Model file for the job. Use its own axes, mm. A direction names the side the tool comes from. Coordinates: 2 decimals unless noted, no trailing zeros. Order: outer loops, then holes, each group sorted by start corner. A loop starts at its lowest first (then second) coordinate and runs counter-clockwise, first axis right, second up. Notation, with made-up numbers: (64.5, 5.25) -> (73.5, 5.25) arc R12 ccw to (73.5, 10.25) -> close; hole circle Ø10 at (-18.5, 11.5). An arc over 180 degrees is marked (long way). Use CSV: the item, a comma, the result in double quotes. Start each with the question number.
(1) Cut at C-C on x = 21. Write the cut outline in (y, z), plus the area to 3 significant figures.
(2) Pin check, flat tips, straight feed: pin 1 Ø1 at (x, z) = (13.5, 0) entering from -Y; pin 2 Ø0.5 at (x, y) = (0.5, 0.5) entering from +Z; pin 3 Ø3 at (x, y) = (21, -1) entering from +Z; pin 4 Ø1 at (y, z) = (-2, 0.5) entering from +X. Stop position of each tip, or through.
(3) Cut at D-D on x = 33.5. Write the cut outline in (y, z) (3 decimals).
(4) Probe L1, parallel to X at y = -1.5, z = 0.15; L2, parallel to X at y = 1.7, z = 0.35; L3, parallel to Y at x = 20, z = 0.15 (3 decimals). List the from-to ranges inside material, lowest first.
(5) Cut at B-B on z = 0. Write the cut outline in (x, y) (3 decimals).
(6) Pull direction Z, two halves, no side cores. Call faces 1 (the flat face through (32, 2, 0)), 2 (the cylindrical face through (0.99, -0.65, 2.93)), 3 (the flat face through (0.5, 0, 1)): pulls with the +Z half, pulls with the -Z half, needs draft (parallel to the pull), parting line crosses it, or undercut.
(7) Cut at A-A on y = 0. Write the cut outline in (x, z) (3 decimals), plus the area to 3 significant figures.
(8) Tool access for faces 4 (the flat face through (0, 0, 2)), 5 (the flat face through (1, 0, 0)), 6 (the cylindrical face through (34.22, -1.29, 0.99)): list every direction of +Z, -Z, +X, -X, +Y, -Y with a clear straight run to the whole face (end or side of a thin tool).
Autodesk Inventor part; units mm, degrees
ref_plane "YZ Plane" through (0, 0, 0) normal (1, 0, 0) x (0, 1, 0)
ref_plane "XZ Plane" through (0, 0, 0) normal (0, 1, 0) x (-1, 0, 0)
ref_plane "XY Plane" through (0, 0, 0) normal (0, 0, 1) x (1, 0, 0)
sketch "Sketch1" plane through (0, 0, 0) normal (0, 0, 1) x (1, 0, 0)
  line L0 (0, 0) -> (2, 0)
  line L1 (2, 0) -> (2, 3)
  line L2 (2, 3) -> (0, 3)
  line L3 (0, 3) -> (0, 0)
  line L4 (2, 0) -> (32, 0)
  line L5 (32, 0) -> (32, 2.25)
  line L6 (32, 2.25) -> (2, 2.25)
  line L7 (2, 2.25) -> (2, 0)
  line L8 (32, 0) -> (36.5, 0)
  line L9 (36.5, 0) -> (36.5, 1.625)
  line L10 (36.5, 1.625) -> (32, 1.625)
  line L11 (32, 1.625) -> (32, 0)
  dimension "d0" = 36.5
  dimension "d1" = 32
  dimension "d2" = 2
  dimension "d3" = 6
  dimension "d4" = 4.5
  dimension "d5" = 3.25
revolve "Revolution1" add sketch "Sketch1" angle 360 about axis through (2, 0, 0) along (1, 0, 0)
sketch "Sketch2" plane through (0, 0, 0) normal (0, 1, 0) x (-1, 0, 0)
  line L0 (0, 3) -> (0, -3)
  line L1 (-2, 3) -> (-2, -3)
  line L2 (0, 1) -> (-1, 1)
  line L3 (-1, 1) -> (-1, -1)
  line L4 (-1, -1) -> (0, -1)
  line L5 (0, -1) -> (0, 1)
  dimension "d10" = 2
  dimension "d11" = 2
  dimension "d12" = 2
  dimension "d15" = 1
extrude "Extrusion1" cut sketch "Sketch2" along normal mid plane 10
thread "Thread1"
equation "\"d11\" = d12"
properties part number "406-02" material "Steel, Mild"
Outcome:
1,outline,"circle Ø4.5 at (0, 0)"
1,area,"15.9 mm2"
2,pin 1,"y = -2.25"
2,pin 2,"z = 2.99"
2,pin 3,"z = 2.25"
2,pin 4,"x = 36.5"
3,outline,"circle Ø3.25 at (0, 0)"
4,L1,"1 to 36.5"
4,L2,"1 to 32"
4,L3,"-2.245 to 2.245"
5,outline,"(1, -3) -> (2, -3) -> (2, -2.25) -> (32, -2.25) -> (32, -1.625) -> (36.5, -1.625) -> (36.5, 1.625) -> (32, 1.625) -> (32, 2.25) -> (2, 2.25) -> (2, 3) -> (1, 3) -> close"
6,face 1,"needs draft"
6,face 2,"parting line crosses it"
6,face 3,"undercut"
7,outline,"(0, -3) -> (2, -3) -> (2, -2.25) -> (32, -2.25) -> (32, -1.625) -> (36.5, -1.625) -> (36.5, 1.625) -> (32, 1.625) -> (32, 2.25) -> (2, 2.25) -> (2, 3) -> (0, 3) -> (0, 1) -> (1, 1) -> (1, -1) -> (0, -1) -> close"
7,area,"160 mm2"
8,face 4,"+Z, -Z, -X, +Y, -Y"
8,face 5,"-X, +Y, -Y"
8,face 6,"+X"
